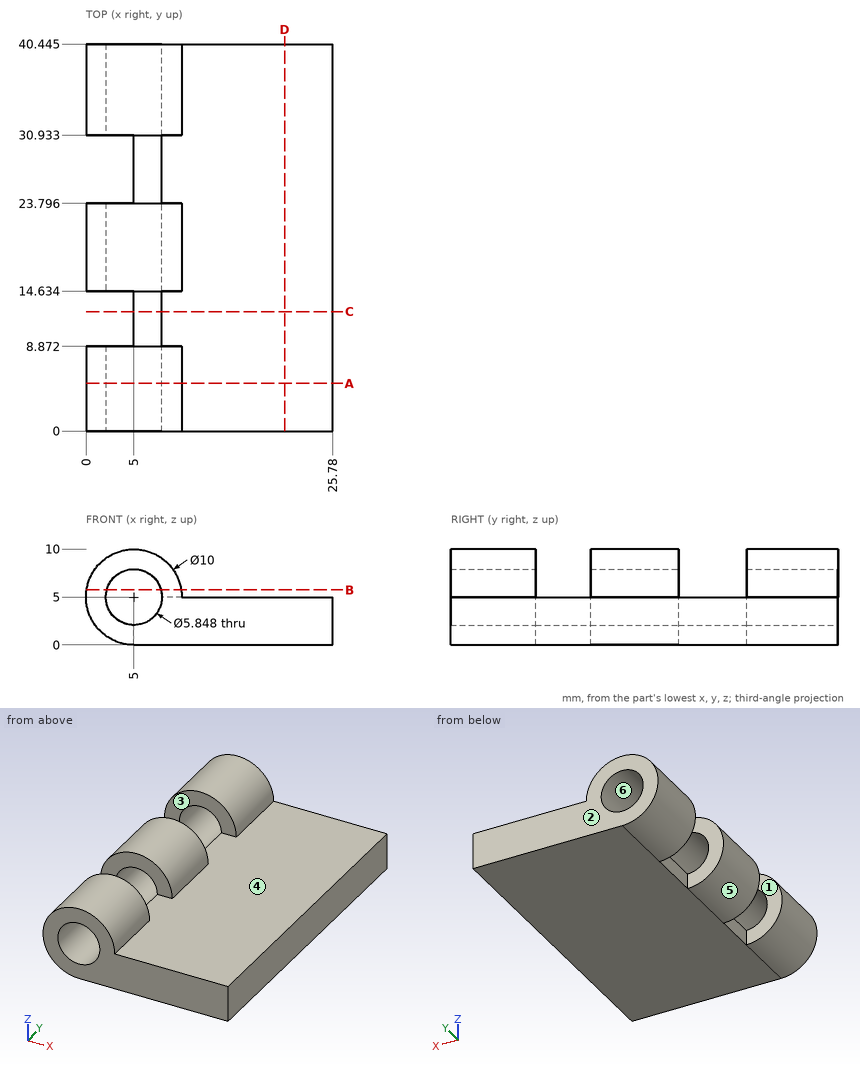
Source: three-view drawing plus pictorial views. Frame: mm from the lowest corner of the part. A direction names the side the tool comes from. Coordinates: 2 decimals unless noted, no trailing zeros. Order: outer loops, then holes, each group sorted by start corner. A loop starts at its lowest first (then second) coordinate and runs counter-clockwise, first axis right, second up.
Item 1: Cut plane A-A (y = 5). Return loops of the section in (x, z), plus the area to 3 significant figures.
Output values:
outline: (5, 0) - (25.78, 0) - (25.78, 5) - (10, 5) arc R5 ccw (long way) to start; hole circle Ø5.85 at (5, 5)
area: 136 mm2
Item 2: Pull-direction query (Z, two-part tool) for the marked faces 3, 4, 5 and 6; classes: pulls with the +Z half, pulls with the -Z half, needs draft (parallel to the pull), parting line crosses it, or undercut.
Output values:
face 3: needs draft
face 4: pulls with the +Z half
face 5: parting line crosses it
face 6: undercut
Item 3: Cut plane C-C (y = 12.5). Return loops of the section in (x, z).
Output values:
outline: (5, 0) - (25.78, 0) - (25.78, 5) - (7.92, 5) arc R2.92 cw to (5, 2.08) - close
Item 4: First-contact query: P1, Ø1.7, axis at y = 11, z = 1.5, coming from the -X side; P2, Ø2, axis at y = 21.5, z = 3.5, coming from the -X side (1 decimal); P3, Ø4, axis at x = 7, y = 26, coming from the +Z side. Flat tips, straight axial feed; report the tip coordinate or a pass-through.
Output values:
P1: stops at x = 5
P2: stops at x = 0
P3: stops at z = 5
Item 5: Set-up query: the marked faces 1 and 2. Return all of +Z, -Z, +X, -X, +Y, -Y with unobstructed straight access to the full face (end or side cutting, diameter ignored); none if empty.
Output values:
face 1: +Z, -X
face 2: +Z, -Z, +X, -X, +Y
Item 6: Cut plane D-D (x = 20.75). Return loops of the section in (y, z) (1 decimal).
Output values:
outline: (0, 0) - (40.4, 0) - (40.4, 5) - (0, 5) - close
Item 7: Material intervals for line 1 (Y direction, x = 9.5, z = 6.75) (1 decimal); line 2 (Z direction, x = 5, y = 17.5); line 3 (Z direction, x = 23.75, y = 18), sorted ascending.
Output values:
line 1: y = 0 to 8.9, 14.6 to 23.8, 30.9 to 40.4
line 2: z = 0 to 2.08, 7.92 to 10
line 3: z = 0 to 5
Item 8: Cut plane B-B (z = 5.75). Return loops of the section in (x, y) (1 decimal), plus the area to 3 significant figures.
Output values:
outline: (0.1, 0) - (2.2, 0) - (2.2, 8.9) - (0.1, 8.9) - close; (0.1, 14.6) - (2.2, 14.6) - (2.2, 23.8) - (0.1, 23.8) - close; (0.1, 30.9) - (2.2, 30.9) - (2.2, 40.4) - (0.1, 40.4) - close; (7.8, 0) - (9.9, 0) - (9.9, 8.9) - (7.8, 8.9) - close; (7.8, 14.6) - (9.9, 14.6) - (9.9, 23.8) - (7.8, 23.8) - close; (7.8, 30.9) - (9.9, 30.9) - (9.9, 40.4) - (7.8, 40.4) - close
area: 117 mm2
